Input: part model. Units: mm. Frame: model coordinates. A direction names the side the tool comes from. Give positions to 0.01 mm unless a question says otherwise; leave off trailing zeros. Loops run counter-clockwise (first coordinate to the right, second up) from the corner with the lowest first, then second, coordinate; pieces in that order, holes last. Notation, with made-up numbers: (24, -4.5) - (38, -4.5) arc R24 cw to (38, 25.5) - close; hole circle Ø10 at (63.25, 20). An arc over 180 degrees is marked (long way). One line per item, written item: value.
from build123d import *

# Parameters (mm, degrees)
SKETCH1_R           = 50.8
BOSS_EXTRUDE1_DEPTH = 25.4
SKETCH2_R           = 76.2
BOSS_EXTRUDE2_DEPTH = 89.9
SKETCH4_R           = 76.2
BOSS_EXTRUDE3_DEPTH = 86
CUT_EXTRUDE1_START  = -166.1000001
CUT_EXTRUDE1_DEPTH  = 152.4000001
SKETCH7_R           = 50.8
CUT_EXTRUDE2_DEPTH  = 25.4


# Read off the part's stored shape, not the designer's step: Cut-Extrude1
with BuildPart() as part:
    # Sketch1 → Boss-Extrude1 (new body)
    with BuildSketch(Plane(origin=(0, 0, 0), x_dir=(1, 0, 0), z_dir=(0, 1, 0))):
        with Locations(Location((0, 0, 0), (0, 0, 270))):
            Circle(SKETCH1_R)
    extrude(amount=BOSS_EXTRUDE1_DEPTH)

    # Sketch2 → Boss-Extrude2 (add)
    with BuildSketch(Plane(origin=(0, 25.4, 0), x_dir=(1, 0, 0), z_dir=(0, 1, 0))):
        with Locations(Location((0, 0, 0), (0, 0, 270))):
            Circle(SKETCH2_R)
    extrude(amount=BOSS_EXTRUDE2_DEPTH)

    # Sketch4 → Boss-Extrude3 (add, symmetric)
    with BuildSketch(Plane(origin=(0, 0, 0), x_dir=(0, 0, -1), z_dir=(1, 0, 0))):
        with Locations((0, 115.3)):
            Circle(SKETCH4_R)
    extrude(amount=BOSS_EXTRUDE3_DEPTH, both=True)

    # Cut-Extrude1 outline → Cut-Extrude1 (cut)
    with BuildSketch(Plane.XZ.offset(-25.4).offset(CUT_EXTRUDE1_START)):
        with BuildLine():
            Line((0, 76.2), (0, 148.473309088))
            ThreePointArc((0, 148.473309088), (-148.473309088, 0), (0, -148.473309088))
            Line((0, -148.473309088), (0, -76.2))
            ThreePointArc((0, -76.2), (-76.2, 0), (0, 76.2))
        make_face()
    extrude(amount=CUT_EXTRUDE1_DEPTH, mode=Mode.SUBTRACT)

    # Sketch7 → Cut-Extrude2 (cut)
    with BuildSketch(Plane(origin=(86, 0, 0), x_dir=(0, 0, -1), z_dir=(1, 0, 0))):
        with Locations((0, 115.3)):
            Circle(SKETCH7_R)
    extrude(amount=-CUT_EXTRUDE2_DEPTH, mode=Mode.SUBTRACT)


solid = part.part
Item 1: Section C-C, the plane x = 0. Output: boundary loops of the cut face in (y, z), and give its area (3 significant figures).
Verdict:
outline: (0, -50.8) - (25.4, -50.8) - (25.4, -76.2) - (115.3, -76.2) arc R76.2 ccw to (115.3, 76.2) - (25.4, 76.2) - (25.4, 50.8) - (0, 50.8) - close
area: 25,400 mm^2
Item 2: Section A-A, the plane y = 115.3. Output: boundary loops of the cut face in (x, z).
Verdict:
outline: (0, -76.2) - (86, -76.2) - (86, -50.8) - (60.6, -50.8) - (60.6, 50.8) - (86, 50.8) - (86, 76.2) - (0, 76.2) arc R76.2 ccw to start
Item 3: Access query for faces 4 (the face through (1, 0, -1)), 5 (the face through (-30.911, 12.522, -40.313)), 6 (the face through (60.6, 116, 1)). Directions: +Z, -Z, +X, -X, +Y, -Y. A direction counts if a zero-diameter tool reaches every point of the face in a straight line with its end or side. Return the directions, or none.
Verdict:
face 4: +Z, -Z, +X, -X, -Y
face 5: -Y
face 6: +X
Item 4: Section D-D, the plane y = 14. Output: boundary loops of the cut face in (x, z), and give its area (3 significant figures).
Verdict:
outline: circle Ø101.6 at (0, 0)
area: 8,110 mm^2
Item 5: Draft query along Y for faces 1 (the face through (86, 99, -50)), 2 (the face through (24.06, 190.85, 9.92)), 3 (the face through (73.478, 65.708, 11.012)). Return one class per face: pulls with the +Y half, pulls with the -Y half, needs draft (parallel to the pull), parting line crosses it, or undercut.
Verdict:
face 1: needs draft
face 2: parting line crosses it
face 3: undercut
Item 6: Section B-B, the plane z = 0. Output: boundary loops of the cut face in (x, y), and give its area (3 significant figures).
Verdict:
outline: (-76.2, 25.4) - (-50.8, 25.4) - (-50.8, 0) - (50.8, 0) - (50.8, 25.4) - (76.2, 25.4) - (76.2, 39.1) - (86, 39.1) - (86, 64.5) - (60.6, 64.5) - (60.6, 166.1) - (86, 166.1) - (86, 191.5) - (-76.2, 191.5) - close
area: 26,800 mm^2
Item 7: Material intervals for L1, parallel to Y at x = 73.5, z = 0; L2, parallel to Z at x = 69, y = 115; L3, parallel to Y at x = 78, z = 0, sorted ascending.
Verdict:
L1: y = 25.4 to 64.5, 166.1 to 191.5
L2: z = -76.2 to -50.8, 50.8 to 76.2
L3: y = 39.1 to 64.5, 166.1 to 191.5
Item 8: Pin query (flat end, axial travel): P1, Ø10, axis at x = 24, z = -36, coming from the +Y side; P2, Ø4, axis at x = 42.5, z = -47.5, coming from the -Y side; P3, Ø1.5, axis at y = 26.5, z = -11, coming from the +X side; P4, Ø10, axis at x = -57, z = -59.5, coming from the +Y side. Return the tip coordinate at first contact, or that it passes through.
Verdict:
P1: stops at y = 184.91
P2: stops at y = 25.4
P3: stops at x = 75.51
P4: passes through
